from build123d import *

# Parameters (mm, degrees)
SKETCH_W   = 21
SKETCH_H   = 24
SKETCH_R   = 1.3
SKETCH_R_2 = 5
PAD_DEPTH  = 3
FILLET_R   = 1


with BuildPart() as part:
    # Sketch → Pad (new body)
    with BuildSketch(Plane.XY):
        with Locations((10.5, 12)):
            Rectangle(SKETCH_W, SKETCH_H)
        with Locations((2.5, 17)):
            Circle(SKETCH_R, mode=Mode.SUBTRACT)
        with Locations((18.5, 17)):
            Circle(SKETCH_R, mode=Mode.SUBTRACT)
        with Locations((2.5, 7)):
            Circle(SKETCH_R, mode=Mode.SUBTRACT)
        with Locations((18.5, 7)):
            Circle(SKETCH_R, mode=Mode.SUBTRACT)
        with Locations((10.5, 12)):
            Circle(SKETCH_R_2, mode=Mode.SUBTRACT)
    extrude(amount=PAD_DEPTH)

    # Fillet
    fillet_edges = [part.edges().sort_by_distance(p)[0] for p in [
        (0, 0, 1.5),
        (21, 0, 1.5),
        (21, 24, 1.5),
        (0, 24, 1.5),
    ]]
    fillet(fillet_edges, radius=FILLET_R)


solid = part.part
Build history of the part. All positions in model axes, mm. Give positions to 0.01 mm unless a question says otherwise; leave off trailing zeros. Loops run counter-clockwise (first coordinate to the right, second up) from the corner with the lowest first, then second, coordinate; pieces in that order, holes last. Notation, with made-up numbers: (-10.75, -4) - (23.25, -4) arc R28 cw to (23.25, 24) - close; hole circle Ø8 at (-19, -35.5). An arc over 180 degrees is marked (long way). Write item = value, one per line. Start each with the question number.
1) Band-saw the part on D-D on x = 6.25. Give the cut face in (y, z).
2) Pull direction Y, two halves, no side cores. Call faces 1 (the cylindrical face through (20.699, 23.715, 1.521)), 2 (the flat face through (0, 12, 1)), 3 (the cylindrical face through (2.22, 5.73, 1.48)): +Y half, -Y half, draft (parallel to the pull), parting line (faces both ways), or undercut.
3) Band-saw the part on B-B on x = 18.5. Give the cut face in (y, z), plus the area to 3 significant figures.
4) Band-saw the part on C-C on y = 14.5. Give the cut face in (x, z).
5) Probe probe 1 along Y at (x, z) = (18.5, 0.2); probe 2 along X at (y, z) = (7.5, 1.75); probe 3 along Y at (x, z) = (10.5, 2.1). List the from-to ranges inside material, lowest first. Write a range as from..to.
6) Band-saw the part on A-A on z = 2.1. Give the cut face in (x, y).
7) Drop a flat-ended pin along its axis: pin 1 Ø2 at (x, y) = (18.5, 17) entering from +Z. Give the stop position or say it passes through.
Final values:
q1.outline = (0, 0) - (9.37, 0) - (9.37, 3) - (0, 3) - close; (14.63, 0) - (24, 0) - (24, 3) - (14.63, 3) - close
q2.face_1 = +Y half
q2.face_2 = draft
q2.face_3 = undercut
q3.outline = (0, 0) - (5.7, 0) - (5.7, 3) - (0, 3) - close; (8.3, 0) - (15.7, 0) - (15.7, 3) - (8.3, 3) - close; (18.3, 0) - (24, 0) - (24, 3) - (18.3, 3) - close
q3.area = 56.4 mm²
q4.outline = (0, 0) - (6.17, 0) - (6.17, 3) - (0, 3) - close; (14.83, 0) - (21, 0) - (21, 3) - (14.83, 3) - close
q5.probe_1 = 0..5.7, 8.3..15.7, 18.3..24
q5.probe_2 = 0..1.3, 3.7..8.32, 12.68..17.3, 19.7..21
q5.probe_3 = 0..7, 17..24
q6.outline = (0, 1) arc R1 ccw to (1, 0) - (20, 0) arc R1 ccw to (21, 1) - (21, 23) arc R1 ccw to (20, 24) - (1, 24) arc R1 ccw to (0, 23) - close; hole circle Ø2.6 at (2.5, 7); hole circle Ø2.6 at (2.5, 17); hole circle Ø10 at (10.5, 12); hole circle Ø2.6 at (18.5, 7); hole circle Ø2.6 at (18.5, 17)
q7.pin_1 = through
